For this review, take the finished solid that the model builds, in its own axes (mm). Face numbers are marked on the shaded views. A direction names the side the tool comes from. Round coordinates to 2 decimals unless told otherwise and drop trailing zeros. Order: outer loops, then holes, each group sorted by start corner. A loop starts at its lowest first (then second) coordinate and runs counter-clockwise, first axis right, second up. Notation, with made-up numbers: (77.5, 37.25) - (106.5, 37.25) arc R9 ccw to (106.5, 41.25) - close; hole circle Ø4 at (-13, -36.5). An arc over 180 degrees is marked (long way). One line per item, written item: value.
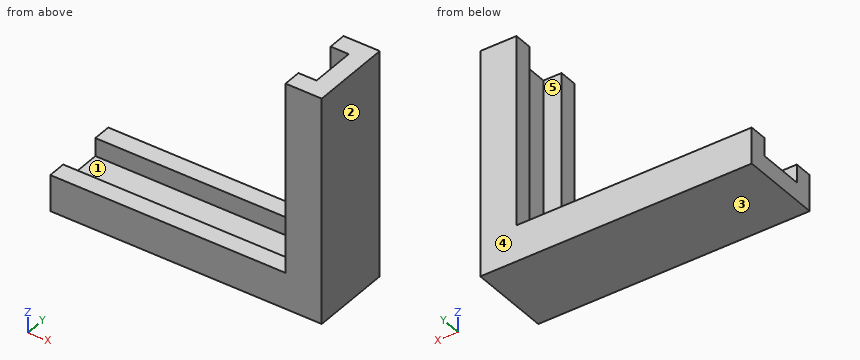
```python
from build123d import *

# Parameters (mm, degrees)
F0_W     = 2
F0_H     = 5
F0_W_2   = 26
F0_H_2   = 2
F1_DEPTH = 2
F2_DEPTH = 4
F3_DEPTH = 25


with BuildPart() as f1:
    # F0 (on Top) → F1 (new body)
    with BuildSketch(Plane.XY):
        Polygon((11, -4.5), (15, -4.5), (15, -2.5), (13, -2.5), (11, -2.5), align=None)
        Polygon((-15, -4.5), (11, -4.5), (11, -2.5), (-13.6096680164, -2.5), (-15, -2.5), align=None)
        with Locations((14, 0)):
            Rectangle(F0_W, F0_H)
        with Locations((12, 0)):
            Rectangle(F0_W, F0_H)
        Polygon((-13.6096680164, -2.5), (11, -2.5), (11, 2.5), (-15, 2.5), (-15, -2.5), align=None)
        Polygon((13, 2.5), (15, 2.5), (15, 4.5), (11, 4.5), (11, 2.5), align=None)
        with Locations((-2, 3.5)):
            Rectangle(F0_W_2, F0_H_2)
    extrude(amount=F1_DEPTH)

    # F0 (on Top) → F2 (join)
    with BuildSketch(Plane.XY):
        Polygon((11, -4.5), (15, -4.5), (15, -2.5), (13, -2.5), (11, -2.5), align=None)
        Polygon((-15, -4.5), (11, -4.5), (11, -2.5), (-13.6096680164, -2.5), (-15, -2.5), align=None)
        with Locations((14, 0)):
            Rectangle(F0_W, F0_H)
        Polygon((13, 2.5), (15, 2.5), (15, 4.5), (11, 4.5), (11, 2.5), align=None)
        with Locations((-2, 3.5)):
            Rectangle(F0_W_2, F0_H_2)
    extrude(amount=F2_DEPTH)

    # F0 (on Top) → F3 (join)
    with BuildSketch(Plane.XY):
        with Locations((14, 0)):
            Rectangle(F0_W, F0_H)
        Polygon((11, -4.5), (15, -4.5), (15, -2.5), (13, -2.5), (11, -2.5), align=None)
        Polygon((13, 2.5), (15, 2.5), (15, 4.5), (11, 4.5), (11, 2.5), align=None)
    extrude(amount=F3_DEPTH)


solid = f1.part
```
Item 1: Take a section at A-A (z = 12.5). Write out the cut boundary in (x, y), plus the area to 3 significant figures.
Returned:
outline: (11, -4.5) - (15, -4.5) - (15, 4.5) - (11, 4.5) - (11, 2.5) - (13, 2.5) - (13, -2.5) - (11, -2.5) - close
area: 26.0 mm^2
Item 2: The part is to be moulded in two halves that separate along Y. For the marked faces 3, 4 and 5, say which applies: +Y half, -Y half, draft (parallel to the pull), parting line (faces both ways), or undercut.
Returned:
face 3: draft
face 4: +Y half
face 5: undercut
Item 3: Wall thickness on line 1 (Y direction, x = 12.5, z = 14.5); line 2 (X direction, y = 2.25, z = 6.75); line 3 (Z direction, x = -2.5, y = -1.75): over which ranges is each line inside the solid? List them lowest first.
Returned:
line 1: -4.5 to -2.5, 2.5 to 4.5
line 2: 13 to 15
line 3: 0 to 2
Item 4: Take a section at D-D (y = -1.75). Write out the cut boundary in (x, z).
Returned:
outline: (-15, 0) - (15, 0) - (15, 25) - (13, 25) - (13, 2) - (-15, 2) - close
Item 5: For P1, Ø1, axis at x = 4.5, y = 1.5, coming from the +Z side; P2, Ø11.5, axis at x = -5.5, z = 8.5, coming from the -Y side; P3, Ø1.6, axis at x = -3.5, y = -3.5, coming from the +Z side; P4, Ø0.6, axis at y = -3.5, z = 17, coming from the -X side, all flat-tipped, find the tip position at first contact; note any pin that passes through.
Returned:
P1: z = 2
P2: y = -4.5
P3: z = 4
P4: x = 11
Item 6: Machinability: for the marked faces 1 and 2, which of the approach directions +Z, -Z, +X, -X, +Y, -Y give a long, thin tool a straight path to every point of the face, cutting with its end or side? Answer none if there is none.
Returned:
face 1: +Z, -X
face 2: +Z, -Z, +X, +Y, -Y
Item 7: Take a section at B-B (y = 3). Write out the cut boundary in (x, z), plus the area to 3 significant figures.
Returned:
outline: (-15, 0) - (15, 0) - (15, 25) - (11, 25) - (11, 4) - (-15, 4) - close
area: 204 mm^2
Item 8: Take a section at C-C (x = -10). Write out the cut boundary in (y, z).
Returned:
outline: (-4.5, 0) - (4.5, 0) - (4.5, 4) - (2.5, 4) - (2.5, 2) - (-2.5, 2) - (-2.5, 4) - (-4.5, 4) - close
